Could you check a few things on this model? Use its own coordinates, in mm. A direction names the side the tool comes from. Give positions to 0.01 mm unless a question says otherwise; leave off trailing zeros. Order: outer loops, then holes, each group sorted by start corner. A loop starts at its lowest first (then second) coordinate and runs counter-clockwise, first axis right, second up. Notation, with made-up numbers: M 48.25,75.5 L 63.25,75.5 A30 ccw 63.25,97.5 Z; hole C 79.5,-39.5 d11. An arc over 180 degrees is marked long. Answer in a Markdown table with one row per item. Add a question column.
```python
from build123d import *

# Parameters (mm, degrees)
SKETCH1_W             = 36
SKETCH1_H             = 36
BOSS_EXTRUDE1_DEPTH   = 15
SHELL1_T              = 3
CUT_EXTRUDE1_REACH    = 52.289
SKETCH2_W             = 25
SKETCH2_H             = 11
CUT_EXTRUDE2_REACH    = 52.289
SKETCH3_W             = 18
SKETCH3_H             = 9
CUT_EXTRUDE3_REACH    = 36.728
SKETCH5_W             = 29
SKETCH5_H             = 29
FILLET1_R             = 2
CUT_EXTRUDE4_REACH    = 52.289
SKETCH6_W             = 22
SKETCH6_H             = 14
FILLET2_R             = 1
SKETCH9_W             = 12
SKETCH9_H             = 10
BOSS_EXTRUDE3_DEPTH   = 5
BOSS_EXTRUDE4_DEPTH   = 10
SKETCH11_R            = 1.5
CUT_EXTRUDE5_DEPTH    = 5
CUT_EXTRUDE6_REACH    = 43.219
SKETCH12_R            = 3
CUT_EXTRUDE7_REACH    = 45.058
MIRROR3_OUTLINE_R     = 1.5
MIRROR3_DEPTH         = 5
MIRROR3_START         = 5
MIRROR3_2_OUTLINE_R   = 3
MIRROR3_2_DEPTH       = 13
MIRROR3_START_2       = 27.639914186
MIRROR3_3_OUTLINE_W   = 20
MIRROR3_3_OUTLINE_H   = 12
MIRROR3_3_OUTLINE_H_2 = 11
MIRROR3_3_DEPTH       = 9.360085814
CHAMFER1_SIZE         = 2
FILLET3_R             = 1


with BuildPart() as part:
    # Sketch1 → Boss-Extrude1 (new body)
    with BuildSketch(Plane(origin=(0, 0, 0), x_dir=(1, 0, 0), z_dir=(0, 1, 0))):
        Rectangle(SKETCH1_W, SKETCH1_H)
    extrude(amount=BOSS_EXTRUDE1_DEPTH)

    # Shell1
    shell1_openings = [part.faces().sort_by_distance(p)[0] for p in [
        (0, 0, 0),
    ]]
    offset(amount=SHELL1_T, openings=shell1_openings, kind=Kind.INTERSECTION)

    # Sketch2 → Cut-Extrude1 (cut, up to next)
    with BuildSketch(Plane.XY.offset(21), mode=Mode.PRIVATE) as cut_extrude1_sk1:
        with Locations((0, 5.5)):
            Rectangle(SKETCH2_W, SKETCH2_H)
    cut_extrude1_tool1 = extrude(cut_extrude1_sk1.sketch, amount=-CUT_EXTRUDE1_REACH, mode=Mode.PRIVATE) & part.part
    add(cut_extrude1_tool1.solids().sort_by_distance((0, 5.5, 21))[0], mode=Mode.SUBTRACT)

    # Sketch3 → Cut-Extrude2 (cut, up to next)
    with BuildSketch(Plane(origin=(21, 0, 0), x_dir=(0, 0, -1), z_dir=(1, 0, 0)), mode=Mode.PRIVATE) as cut_extrude2_sk1:
        with Locations((-2, 4.5)):
            Rectangle(SKETCH3_W, SKETCH3_H)
    cut_extrude2_tool1 = extrude(cut_extrude2_sk1.sketch, amount=-CUT_EXTRUDE2_REACH, mode=Mode.PRIVATE) & part.part
    add(cut_extrude2_tool1.solids().sort_by_distance((21, 4.5, 2))[0], mode=Mode.SUBTRACT)

    # Sketch5 → Cut-Extrude3 (cut, up to next)
    with BuildSketch(Plane(origin=(0, 18, 0), x_dir=(1, 0, 0), z_dir=(0, 1, 0)), mode=Mode.PRIVATE) as cut_extrude3_sk1:
        Rectangle(SKETCH5_W, SKETCH5_H)
    cut_extrude3_tool1 = extrude(cut_extrude3_sk1.sketch, amount=-CUT_EXTRUDE3_REACH, mode=Mode.PRIVATE) & part.part
    add(cut_extrude3_tool1.solids().sort_by_distance((0, 18, 0))[0], mode=Mode.SUBTRACT)

    # Fillet1
    fillet1_edges = [part.edges().sort_by_distance(p)[0] for p in [
        (14.5, 16.5, -14.5),
        (14.5, 16.5, 14.5),
        (-14.5, 16.5, 14.5),
        (-14.5, 16.5, -14.5),
    ]]
    fillet(fillet1_edges, radius=FILLET1_R)

    # Sketch6 → Cut-Extrude4 (cut, up to next)
    with BuildSketch(Plane(origin=(0, 0, -21), x_dir=(-1, 0, 0), z_dir=(0, 0, -1)), mode=Mode.PRIVATE) as cut_extrude4_sk1:
        with Locations((0, 7)):
            Rectangle(SKETCH6_W, SKETCH6_H)
    cut_extrude4_tool1 = extrude(cut_extrude4_sk1.sketch, amount=-CUT_EXTRUDE4_REACH, mode=Mode.PRIVATE) & part.part
    add(cut_extrude4_tool1.solids().sort_by_distance((0, 7, -21))[0], mode=Mode.SUBTRACT)

    # Fillet2
    fillet2_edges = [part.edges().sort_by_distance(p)[0] for p in [
        (-11, 14, -19.5),
        (11, 14, -19.5),
        (12.5, 11, 19.5),
        (-12.5, 11, 19.5),
        (19.5, 9, 11),
        (19.5, 9, -7),
    ]]
    fillet(fillet2_edges, radius=FILLET2_R)

    # Sketch9 → Boss-Extrude3 (add)
    with BuildSketch(Plane.XZ):
        with Locations((-27, 16)):
            Rectangle(SKETCH9_W, SKETCH9_H)
    boss_extrude3 = extrude(amount=-BOSS_EXTRUDE3_DEPTH)

    # Sketch10 → Boss-Extrude4 (add)
    with BuildSketch(Plane.XY.offset(21)):
        Polygon((-21, 18), (-33, 5), (-21, 5), align=None)
    boss_extrude4 = extrude(amount=-BOSS_EXTRUDE4_DEPTH)

    # Sketch11 → Cut-Extrude5 (cut)
    with BuildSketch(Plane.XZ):
        with Locations(Location((-28, 16, 0), (0, 0, 270))):
            Circle(SKETCH11_R)
    cut_extrude5 = extrude(amount=-CUT_EXTRUDE5_DEPTH, mode=Mode.SUBTRACT)

    # Cut-Extrude6: up to this plane
    cut_extrude6_end = Plane(origin=(-21, 18, -6.691806013), z_dir=(-0.7348034446274878, 0.678280102733066, 0))
    # Sketch12 → Cut-Extrude6 (cut, up to the surface)
    with BuildSketch(Plane.XZ.offset(-5), mode=Mode.PRIVATE) as cut_extrude6_sk1:
        with Locations(Location((-28, 16, 0), (0, 0, 270))):
            Circle(SKETCH12_R)
    cut_extrude6_tool1 = split(extrude(cut_extrude6_sk1.sketch, amount=-CUT_EXTRUDE6_REACH, mode=Mode.PRIVATE), bisect_by=cut_extrude6_end, keep=Keep.BOTH, mode=Mode.PRIVATE)
    cut_extrude6 = cut_extrude6_tool1.solids().sort_by_distance((-28, 5, 16))[0]
    add(cut_extrude6, mode=Mode.SUBTRACT)

    # Cut-Extrude7: up to this plane
    cut_extrude7_end = Plane(origin=(-21, 18, -6.691806013), z_dir=(-0.7348034446274878, 0.678280102733066, 0))
    # Sketch13 → Cut-Extrude7 (cut, up to the surface)
    with BuildSketch(Plane.XZ, mode=Mode.PRIVATE) as cut_extrude7_sk1:
        with BuildLine():
            ThreePointArc((-33, 16), (-31.535533906, 19.535533906), (-28, 21))
            Line((-28, 21), (-33, 21))
            Line((-33, 21), (-33, 16))
        make_face()
    cut_extrude7_tool1 = split(extrude(cut_extrude7_sk1.sketch, amount=-CUT_EXTRUDE7_REACH, mode=Mode.PRIVATE), bisect_by=cut_extrude7_end, keep=Keep.BOTH, mode=Mode.PRIVATE)
    # Sketch13 → Cut-Extrude7 (cut, up to the surface)
    with BuildSketch(Plane.XZ, mode=Mode.PRIVATE) as cut_extrude7_sk2:
        with BuildLine():
            Line((-33, 11), (-28, 11))
            ThreePointArc((-28, 11), (-31.535533906, 12.464466094), (-33, 16))
            Line((-33, 16), (-33, 11))
        make_face()
    cut_extrude7_tool2 = split(extrude(cut_extrude7_sk2.sketch, amount=-CUT_EXTRUDE7_REACH, mode=Mode.PRIVATE), bisect_by=cut_extrude7_end, keep=Keep.BOTH, mode=Mode.PRIVATE)
    cut_extrude7 = cut_extrude7_tool1.solids().sort_by_distance((-31.88316, 0, 19.88316))[0] + cut_extrude7_tool2.solids().sort_by_distance((-31.88316, 0, 12.11684))[0]
    add(cut_extrude7, mode=Mode.SUBTRACT)

    # Mirror1: Boss-Extrude3, Boss-Extrude4, Cut-Extrude5, Cut-Extrude6, Cut-Extrude7 across plane
    add(boss_extrude3.mirror(Plane.XY))
    add(boss_extrude4.mirror(Plane.XY))
    add(cut_extrude5.mirror(Plane.XY), mode=Mode.SUBTRACT)
    add(cut_extrude6.mirror(Plane.XY), mode=Mode.SUBTRACT)
    add(cut_extrude7.mirror(Plane.XY), mode=Mode.SUBTRACT)

    # Mirror3: read off the stored shape, not the designer's step
    # Mirror3 outline → Mirror3 (add)
    # profile 1 of 2: a face of its own
    with BuildSketch(Plane(origin=(0, 0, 0), x_dir=(1, 0, 0), z_dir=(0, 1, 0))):
        with BuildLine():
            Line((21, 21), (21, 11))
            Line((21, 11), (28, 11))
            ThreePointArc((28, 11), (33, 16), (28, 21))
            Line((28, 21), (21, 21))
        make_face()
        with Locations((28, 16)):
            Circle(MIRROR3_OUTLINE_R, mode=Mode.SUBTRACT)
    # profile 2 of 2: a face of its own
    with BuildSketch(Plane(origin=(0, 0, 0), x_dir=(1, 0, 0), z_dir=(0, 1, 0))):
        with BuildLine():
            Line((28, -11), (21, -11))
            Line((21, -11), (21, -21))
            Line((21, -21), (28, -21))
            ThreePointArc((28, -21), (33, -16), (28, -11))
        make_face()
        with Locations((28, -16)):
            Circle(MIRROR3_OUTLINE_R, mode=Mode.SUBTRACT)
    extrude(amount=MIRROR3_DEPTH)

    # Mirror3 2 outline → Mirror3 2 (add)
    # profile 1 of 2: a face of its own
    with BuildSketch(Plane(origin=(0, 0, 0), x_dir=(1, 0, 0), z_dir=(0, 1, 0)).offset(MIRROR3_START)):
        with BuildLine():
            Line((21, 21), (21, 11))
            Line((21, 11), (28, 11))
            ThreePointArc((28, 11), (33, 16), (28, 21))
            Line((28, 21), (21, 21))
        make_face()
        with Locations((28, 16)):
            Circle(MIRROR3_2_OUTLINE_R, mode=Mode.SUBTRACT)
    # profile 2 of 2: a face of its own
    with BuildSketch(Plane(origin=(0, 0, 0), x_dir=(1, 0, 0), z_dir=(0, 1, 0)).offset(MIRROR3_START)):
        with BuildLine():
            Line((28, -11), (21, -11))
            Line((21, -11), (21, -21))
            Line((21, -21), (28, -21))
            ThreePointArc((28, -21), (33, -16), (28, -11))
        make_face()
        with Locations((28, -16)):
            Circle(MIRROR3_2_OUTLINE_R, mode=Mode.SUBTRACT)
    extrude(amount=MIRROR3_2_DEPTH)

    # Mirror3 3 outline → Mirror3 3 (cut)
    with BuildSketch(Plane(origin=(0, 0, 0), x_dir=(0.6782801027330657, -0.734803444627488, 0), z_dir=(0.7348034446274879, 0.6782801027330659, 0)).offset(MIRROR3_START_2)):
        with Locations((10, 17)):
            Rectangle(MIRROR3_3_OUTLINE_W, MIRROR3_3_OUTLINE_H)
        with Locations((10, -16.5)):
            Rectangle(MIRROR3_3_OUTLINE_W, MIRROR3_3_OUTLINE_H_2)
    extrude(amount=MIRROR3_3_DEPTH, mode=Mode.SUBTRACT)

    # Chamfer1
    chamfer1_edges = [part.edges().sort_by_distance(p)[0] for p in [
        (-21, 9, 11),
        (-21, 9, -11),
        (21, 9, -11),
    ]]
    chamfer(chamfer1_edges, length=CHAMFER1_SIZE)

    # Fillet3
    fillet3_edges = [part.edges().sort_by_distance(p)[0] for p in [
        (18, 7.5, 18),
        (18, 7.5, -18),
        (-18, 7.5, -18),
        (-18, 7.5, 18),
    ]]
    fillet(fillet3_edges, radius=FILLET3_R)


solid = part.part
```
1. Will these pins go through, and if not, where does the flat tip stop? P1, Ø9, axis at y = 6, z = 3, coming from the -X side; P2, Ø5.5, axis at x = -28, z = -16, coming from the +Y side; P3, Ø5.5, axis at y = 12.5, z = 1, coming from the +X side.
2. For faces 1 (the cylindrical face through (-25, 8, -16)), 2 (the flat face through (23, 7, 11)), 3 (the flat face through (0, 14, -20)), which set-ups out of +Z, -Z, +X, -X, +Y, -Y let a thin tool reach every point of the face, with its end or its side?
3. If I drill on line 1 along Z through (x, y) = (-28, 8); line 2 along Z through (x, y) = (28, 3.55); line 3 along X through (y, z) = (2.9, -16), over which ranges is the centre line in solid material (lowest first)? Write a range as [from, to].
4. Suppose I cut it at A-A on z = 3. List the corners of the cut face in (x, y) for me, plus the area to 3 significant figures.
5. Thinking about a two-plate mould opening in Z: for faces 4 (the flat face through (-18, 7, 0)), 5 (the flat face through (-20, 0, 0)), 6 (the flat face through (21, 13, 1)), which applies, pulls with the +Z half, pulls with the -Z half, needs draft (parallel to the pull), parting line crosses it, or undercut?
Findings below:
| question | item | result |
|---|---|---|
| 1 | P1 | x = -21 |
| 1 | P2 | y = 5 |
| 1 | P3 | x = 21 |
| 2 | face 1 | +Y |
| 2 | face 2 | +X, -Y |
| 2 | face 3 | -Z, -Y |
| 3 | line 1 | [-21, -19], [-13, -11], [11, 13], [19, 21] |
| 3 | line 2 | [-21, -17.5], [-14.5, -11], [11, 14.5], [17.5, 21] |
| 3 | line 3 | [-33, -29.5], [-26.5, -18], [18, 26.5], [29.5, 33] |
| 4 | outline | M -21,0 L -18,0 L -18,15 L -14.5,15 L -14.5,18 L -21,18 Z; M 14.5,15 L 18,15 L 18,9 L 21,9 L 21,18 L 14.5,18 Z |
| 4 | area | 102 mm2 |
| 5 | face 4 | undercut |
| 5 | face 5 | needs draft |
| 5 | face 6 | undercut |
